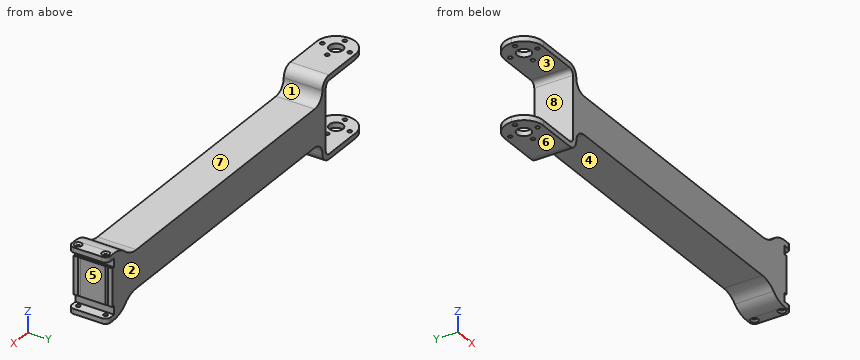
from build123d import *

# Parameters (mm, degrees)
BOSS_EXTRUDE3_DEPTH                                 = 22.6
FILLET2_R                                           = 11.3
BOSS_EXTRUDE4_DEPTH                                 = 22.6
CSK_FOR_M2_COUNTERSUNK_FLAT_HEAD_SCREW1_D           = 2.4
CSK_FOR_M2_COUNTERSUNK_FLAT_HEAD_SCREW1_CSINK_D     = 4.4
CSK_FOR_M2_COUNTERSUNK_FLAT_HEAD_SCREW1_CSINK_ANGLE = 90
FILLET3_R                                           = 3
FILLET3_OF_MIRROR4_R                                = 3
M2_CLEARANCE_HOLE1_D                                = 2.4
M2_CLEARANCE_HOLE1_DEPTH                            = 3
CIRPATTERN1_COUNT                                   = 4
F_8_1_8_1_DIAMETER_HOLE1_D                          = 8.1
F_8_1_8_1_DIAMETER_HOLE1_DEPTH                      = 3
F_8_1_8_1_DIAMETER_HOLE2_D                          = 8.1
M2_CLEARANCE_HOLE2_D                                = 2.4
CIRPATTERN2_COUNT                                   = 4


with BuildPart() as part:
    # Sketch4 → Boss-Extrude3 (new body)
    with BuildSketch(Plane(origin=(0, 0, 0), x_dir=(1, 0, 0), z_dir=(0, 1, 0))):
        with BuildLine():
            Line((0, -21), (0, -24))
            Line((0, -24), (35, -24))
            ThreePointArc((35, -24), (39.242640687, -22.242640687), (41, -18))
            ThreePointArc((41, -18), (43.050252532, -13.050252532), (48, -11))
            Line((48, -11), (230, -11))
            Line((230, -11), (230, 0))
            Line((230, 0), (38, 0))
            Line((38, 0), (38, -18))
            ThreePointArc((38, -18), (37.121320344, -20.121320344), (35, -21))
            Line((35, -21), (0, -21))
        make_face()
    extrude(amount=BOSS_EXTRUDE3_DEPTH)

    # Fillet2
    fillet2_edges = [part.edges().sort_by_distance(p)[0] for p in [
        (0, 0, 22.5),
        (0, 22.6, 22.5),
    ]]
    fillet(fillet2_edges, radius=FILLET2_R - 0.0001)  # a hair under: the kernel refuses the full size

    # Mirror3: part across plane


with BuildPart() as part_1:
    add(part.part)
    add(part.part.mirror(Plane.XY))

    # Sketch5 → Boss-Extrude4 (add, through all)
    with BuildSketch(Plane(origin=(0, 0, 0), x_dir=(1, 0, 0), z_dir=(0, 1, 0))):
        with BuildLine():
            Line((208.5, 11), (228.5, 11))
            Line((228.5, 11), (228.5, 16))
            Line((228.5, 16), (234.6, 16))
            Line((234.6, 16), (234.6, 19))
            Line((234.6, 19), (228.5, 19))
            ThreePointArc((228.5, 19), (223.114835193, 17.962912018), (218.5, 15))
            ThreePointArc((218.5, 15), (213.885164807, 12.037087982), (208.5, 11))
        make_face()
    boss_extrude4 = extrude(amount=BOSS_EXTRUDE4_DEPTH)

    # CSK for M2 Countersunk Flat Head Screw1 (through all)
    with Locations(Plane(origin=(231, 3.3, -19), x_dir=(-1, 0, 0), z_dir=(0, 0, -1))):
        with Locations((0, 0), (0, 16)):
            csk_for_m2_countersunk_flat_head_screw1 = CounterSinkHole(CSK_FOR_M2_COUNTERSUNK_FLAT_HEAD_SCREW1_D / 2, CSK_FOR_M2_COUNTERSUNK_FLAT_HEAD_SCREW1_CSINK_D / 2, counter_sink_angle=CSK_FOR_M2_COUNTERSUNK_FLAT_HEAD_SCREW1_CSINK_ANGLE)

    # Fillet3
    fillet3_edges = [part_1.edges().sort_by_distance(p)[0] for p in [
        (234.6, 0, -17.5),
        (234.6, 22.6, -17.5),
    ]]
    fillet(fillet3_edges, radius=FILLET3_R)

    # Mirror4: Boss-Extrude4, CSK for M2 Countersunk Flat Head Screw1 across plane
    add(boss_extrude4.mirror(Plane.XY))
    add(csk_for_m2_countersunk_flat_head_screw1.mirror(Plane.XY), mode=Mode.SUBTRACT)

    # Fillet3 of Mirror4
    fillet3_of_mirror4_edges = [part_1.edges().sort_by_distance(p)[0] for p in [
        (234.6, 0, 17.5),
        (234.6, 22.6, 17.5),
    ]]
    fillet(fillet3_of_mirror4_edges, radius=FILLET3_OF_MIRROR4_R)

    # M2 Clearance Hole1
    with Locations(Plane(origin=(3.3, 11.3, 24), x_dir=(1, 0, 0), z_dir=(0, 0, 1))):
        with Locations((0, 0)):
            m2_clearance_hole1 = Hole(M2_CLEARANCE_HOLE1_D / 2, depth=M2_CLEARANCE_HOLE1_DEPTH)

    # CirPattern1: M2 Clearance Hole1 ×4 about axis
    cirpattern1_axis = Axis((11.3, 11.3, 0), (0, 0, 1))
    for i in range(1, CIRPATTERN1_COUNT):
        add(m2_clearance_hole1.rotate(cirpattern1_axis, i * 360 / CIRPATTERN1_COUNT), mode=Mode.SUBTRACT)

    # Ø8.1 (8.1) Diameter Hole1
    with Locations(Plane(origin=(11.3, 11.3, -24), x_dir=(-1, 0, 0), z_dir=(0, 0, -1))):
        with Locations((0, 0)):
            Hole(F_8_1_8_1_DIAMETER_HOLE1_D / 2, depth=F_8_1_8_1_DIAMETER_HOLE1_DEPTH)

    # Ø8.1 (8.1) Diameter Hole2 (through all)
    with Locations(Plane(origin=(11.3, 11.3, 24), x_dir=(1, 0, 0), z_dir=(0, 0, 1))):
        with Locations((0, 0)):
            Hole(F_8_1_8_1_DIAMETER_HOLE2_D / 2)

    # M2 Clearance Hole2 (through all)
    with Locations(Plane(origin=(3.3, 11.3, -24), x_dir=(-1, 0, 0), z_dir=(0, 0, -1))):
        with Locations((0, 0)):
            m2_clearance_hole2 = Hole(M2_CLEARANCE_HOLE2_D / 2)

    # CirPattern2: M2 Clearance Hole2 ×4 about axis
    cirpattern2_axis = Axis((11.3, 11.3, 0), (0, 0, 1))
    for i in range(1, CIRPATTERN2_COUNT):
        add(m2_clearance_hole2.rotate(cirpattern2_axis, i * 360 / CIRPATTERN2_COUNT), mode=Mode.SUBTRACT)


solid = part_1.part
Here's how the part is built. I have some questions about the finished solid (model axes, mm). Face numbers are marked on the shaded views. A direction names the side the tool comes from. Coordinates: 2 decimals unless noted, no trailing zeros. Loops run counter-clockwise (first coordinate to the right, second up) from the corner with the lowest first, then second, coordinate; pieces in that order, holes last.
1. For the marked faces 1, 2, 3 and 4, which set-ups out of +Z, -Z, +X, -X, +Y, -Y let a thin tool reach every point of the face, with its end or its side?
2. If we mould it in two halves opening along X, with no side actions, what happens to the marked faces 5, 6, 7 and 8? For each: pulls with the +X half, pulls with the -X half, needs draft (parallel to the pull), parting line crosses it, or undercut.
3. Imagine slicing it at A-A, the plane x = 50. Please give me the cut outline in (y, z), and give its area (3 significant figures).
4. Imagine slicing it at B-B, the plane x = 211. Please give me the cut outline in (y, z).
5. For P1, Ø5, axis at x = 231, y = 6, coming from the +Z side; P2, Ø2, axis at x = 3.3, y = 11.3, coming from the -Z side; P3, Ø1.8, axis at x = 231, y = 7, coming from the -Z side; P4, Ø10, axis at y = 14.5, z = -9.5, coming from the +X side, each with a flat end and sliding along its axis, tell me the tip position at first contact or that it passes through.
6. I need wall thicknesses on L1, parallel to Y at x = 11, z = -22; L2, parallel to Z at x = 11, y = 5; L3, parallel to X at y = 19.3, z = -17.45. Which ranges of each line are inside material? Lowest first, please.
Taken from the geometry:
1. face 1: +Z, +Y, -Y
1. face 2: +Z, -Z, +X, -X, +Y
1. face 3: -X, +Y, -Y
1. face 4: -Z, +Y, -Y
2. face 5: pulls with the +X half
2. face 6: needs draft
2. face 7: undercut
2. face 8: pulls with the -X half
3. outline: (0, -11) - (22.6, -11) - (22.6, 11) - (0, 11) - close
3. area: 497 mm2
4. outline: (0, -11.22) - (22.6, -11.22) - (22.6, 11.22) - (0, 11.22) - close
5. P1: stops at z = 19
5. P2: passes through
5. P3: stops at z = -19
5. P4: stops at x = 230
6. L1: y = 0 to 2.14, 4.46 to 7.26, 15.34 to 18.14, 20.46 to 22.6
6. L2: z = -24 to -21, 21 to 24
6. L3: x = 38 to 41.02, 221.98 to 229.8, 232.2 to 234.6
